Part model, mm, in its own coordinate system. Face numbers are marked on the shaded views. Round coordinates to 2 decimals unless told otherwise and drop trailing zeros. Write each loop counter-clockwise with the first axis right and the second up, starting at its lowest first coordinate (ties: lowest second). Pieces come first, ordered by that corner, then holes. Notation, with made-up numbers: (19, 79.25) -> (75, 79.25) arc R15 cw to (75, 84.25) -> close; hole circle Ø3 at (82, -29). An arc over 180 degrees is marked (long way). Return JSON: item names as keys, results as strings. Group by question number.
```python
from build123d import *

# Parameters (mm, degrees)
SKETCH_1_W             = 224
SKETCH_1_H             = 75
EXTRUDE_1_DEPTH        = 10
CUT_EXTRUDE_1_DEPTH    = 119.533750468
CHAMFER_1_SIZE         = 8
SKETCH_3_W             = 16
SKETCH_3_H             = 17
CUT_EXTRUDE_2_DEPTH    = 119.533750468
CHAMFER_2_SIZE         = 3
PATTERN_LINEAR_1_COUNT = 5
PATTERN_LINEAR_1_PITCH = 24
PATTERN_LINEAR_2_COUNT = 5
PATTERN_LINEAR_2_PITCH = 24


with BuildPart() as part:
    # Эскиз1 → Бобышка-Вытянуть1 (new body)
    with BuildSketch(Plane.XY):
        Rectangle(SKETCH_1_W, SKETCH_1_H)
    extrude(amount=EXTRUDE_1_DEPTH)

    # Эскиз2 → Вырез-Вытянуть1 (cut, symmetric)
    with BuildSketch(Plane.XY.offset(10)):
        with BuildLine():
            Line((-73.5, 4.5), (-73.5, 24.5))
            ThreePointArc((-73.5, 24.5), (-68.5, 29.5), (-63.5, 24.5))
            Line((-63.5, 24.5), (-63.5, 4.5))
            ThreePointArc((-63.5, 4.5), (-68.5, -0.5), (-73.5, 4.5))
        make_face()
    cut_extrude_1 = extrude(amount=CUT_EXTRUDE_1_DEPTH, both=True, mode=Mode.SUBTRACT)

    # Фаска1
    chamfer_1_edges = [part.edges().sort_by_distance(p)[0] for p in [
        (0, -37.5, 0),
    ]]
    chamfer(chamfer_1_edges, length=CHAMFER_1_SIZE)

    # Эскиз3 → Вырез-Вытянуть2 (cut, symmetric)
    with BuildSketch(Plane.XY.offset(10)):
        with Locations((0, -29)):
            Rectangle(SKETCH_3_W, SKETCH_3_H)
    cut_extrude_2 = extrude(amount=CUT_EXTRUDE_2_DEPTH, both=True, mode=Mode.SUBTRACT)

    # Фаска2
    chamfer_2_edges = [part.edges().sort_by_distance(p)[0] for p in [
        (112, 0, 10),
        (-112, 0, 10),
    ]]
    chamfer(chamfer_2_edges, length=CHAMFER_2_SIZE)

    # Линейный массив1: Вырез-Вытянуть2 ×5
    with Locations(*[(-i * PATTERN_LINEAR_1_PITCH, 0, 0) for i in range(1, PATTERN_LINEAR_1_COUNT)]):
        add(cut_extrude_2, mode=Mode.SUBTRACT)

    # Линейный массив2: Вырез-Вытянуть2 ×5
    with Locations(*[(i * PATTERN_LINEAR_2_PITCH, 0, 0) for i in range(1, PATTERN_LINEAR_2_COUNT)]):
        add(cut_extrude_2, mode=Mode.SUBTRACT)

    # Зеркальное отражение2: Вырез-Вытянуть1 across plane
    add(cut_extrude_1.mirror(Plane(origin=(0, 0, 0), x_dir=(0, 0, 1), z_dir=(1, 0, 0))), mode=Mode.SUBTRACT)


solid = part.part
```
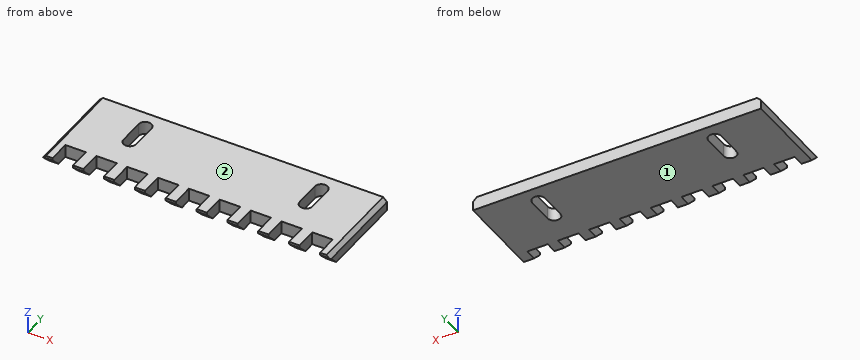
Item 1: Cut at B-B (y = -31.5). State how many separate pieces and enclosed holes the cut face has, then the cut area to 3 significant figures.
Item 2: Flat gauge pin, fed straight in: P1, Ø5, axis at x = 69.5, z = 4.5, coming from the -Y side. Where does the tip first touch, or does it go through?
Item 3: Wall check: L1, parallel to X at y = 8.5, z = 4.5; L2, parallel to Y at x = -68, z = 1.5; L3, parallel to X at y = 20.5, z = 7.25. Give the ranges that are in metal, low to high.
Item 4: Cut at A-A (x = 68.5). Write the cut outline in (y, z), then the cut area to 3 significant figures.
Item 5: Cut at D-D (x = -91). Write the cut outline in (y, z), then the cut area to 3 significant figures.
Item 6: Two-plate mould, pull along Z, no slides. Class the marked faces 1 and 2: released by +Z, released by -Z, zero draft, split by the parting line, or undercut.
Checks:
{
 "1": {"separate pieces": "10", "enclosed holes": "0", "area": "631 mm2"},
 "2": {"P1": "stops at y = -20.5"},
 "3": {"L1": "x = -112 to -73.5, -63.5 to 63.5, 73.5 to 112", "L2": "y = -20.5 to -0.47, 29.47 to 37.5", "L3": "x = -111.75 to -73.5, -63.5 to 63.5, 73.5 to 111.75"},
 "4": {"outline": "(-20.5, 0) -> (-0.5, 0) -> (-0.5, 10) -> (-20.5, 10) -> close; (29.5, 0) -> (37.5, 0) -> (37.5, 10) -> (29.5, 10) -> close", "area": "280 mm2"},
 "5": {"outline": "(-20.5, 0) -> (37.5, 0) -> (37.5, 10) -> (-20.5, 10) -> close", "area": "580 mm2"},
 "6": {"face 1": "released by -Z", "face 2": "released by +Z"}
}
